```python
from build123d import *

# Parameters (mm, degrees)
EXTRUDE1_DEPTH          = 12.7
F_1_4_CLEARANCE_HOLE1_D = 7.14248
CHAMFER1_SIZE           = 4.7625


with BuildPart() as part:
    # Sketch1 → Extrude1 (new, symmetric)
    with BuildSketch(Plane.XY):
        with BuildLine():
            Line((22.225, 26.9875), (0.79375, 26.9875))
            Line((0.79375, 26.9875), (0.79375, 12.675171042))
            ThreePointArc((0.79375, 12.675171042), (0, -12.7), (-0.79375, 12.675171042))
            Line((-0.79375, 12.675171042), (-0.79375, 26.9875))
            Line((-0.79375, 26.9875), (-22.225, 26.9875))
            Line((-22.225, 26.9875), (-22.225, -30.1625))
            Line((-22.225, -30.1625), (-41.275, -30.1625))
            Line((-41.275, -30.1625), (-41.275, -38.1))
            Line((-41.275, -38.1), (41.275, -38.1))
            Line((41.275, -38.1), (41.275, -30.1625))
            Line((41.275, -30.1625), (22.225, -30.1625))
            Line((22.225, -30.1625), (22.225, 26.9875))
        make_face()
    extrude(amount=EXTRUDE1_DEPTH, both=True)

    # 1/4 Clearance Hole1 (through all)
    with Locations(Plane.XZ.offset(38.1)):
        with Locations((-31.75, 0), (31.75, 0)):
            Hole(F_1_4_CLEARANCE_HOLE1_D / 2)

    # Chamfer1
    chamfer1_edges = [part.edges().sort_by_distance(p)[0] for p in [
        (-22.225, 26.9875, 0),
        (22.225, 26.9875, 0),
    ]]
    chamfer(chamfer1_edges, length=CHAMFER1_SIZE)


solid = part.part
```
Can you work these out from the model? Positions are in its coordinate system, mm. A direction names the side the tool comes from. Coordinates: 2 decimals unless noted, no trailing zeros. Loops run counter-clockwise (first coordinate to the right, second up) from the corner with the lowest first, then second, coordinate; pieces in that order, holes last. Notation, with made-up numbers: M -33.5,-12 L -11.5,-12 A8 cw -11.5,-8 Z; hole C 3.25,82.25 d1. An arc over 180 degrees is marked long. Put each result on its own line as item: value. Start each with the question number.
(1) We'd pull the mould along Z, two halves only. Please class faces 5 (the face through (-35.156, -34.076, 1.073)), 6 (the face through (28.344, -34.076, 1.073)), 7 (the face through (-10, -12, 12.7)), 8 (the face through (-41.275, -34, 0)): +Z half, -Z half, draft (parallel to the pull), parting line (faces both ways), or undercut.
(2) Imagine slicing it at C-C on y = 0. List the corners of the cut face in (x, z) for me (3 decimals), and give its area (3 significant figures).
(3) Imagine slicing it at A-A on x = 31.75. List the corners of the cut face in (y, z) for me.
(4) Imagine slicing it at B-B on z = 0. List the corners of the cut face in (x, y) for me (1 decimal).
(5) I need wall thicknesses on probe 1 along Z at (x, y) = (31.75, -35.25); probe 2 along X at (y, z) = (0, -3.5) (3 decimals); probe 3 along X at (y, z) = (13, -4.25) (3 decimals). Which ranges of each line are inside material? Lowest first, please.
(6) Imagine slicing it at D-D on z = -6. List the corners of the cut face in (x, y) for me (1 decimal).
(7) Will these pins go through, and if not, where does the flat tip stop? pin 1 Ø15 at (x, z) = (31.5, -0.5) entering from +Y; pin 2 Ø4 at (y, z) = (18.5, -7.5) entering from +X (3 decimals); pin 3 Ø7 at (y, z) = (22, -5.5) entering from -X (3 decimals).
(8) Which directions (+Z, -Z, +X, -X, +Y, -Y) give clear straight access to the entire face, cutting with the end or side of a thin tool? Please do faces 1 (the face through (22.225, -4, 0)), 2 (the face through (-0.794, 20, 0)), 3 (the face through (-10, -12, -12.7)), 4 (the face through (-22.225, -4, 0)).
Worked answers:
1. face 5: undercut
1. face 6: undercut
1. face 7: +Z half
1. face 8: draft
2. outline: M -22.225,-12.7 L -12.7,-12.7 L -12.7,12.7 L -22.225,12.7 Z; M 12.7,-12.7 L 22.225,-12.7 L 22.225,12.7 L 12.7,12.7 Z
2. area: 484 mm2
3. outline: M -38.1,-12.7 L -30.16,-12.7 L -30.16,-3.57 L -38.1,-3.57 Z; M -38.1,3.57 L -30.16,3.57 L -30.16,12.7 L -38.1,12.7 Z
4. outline: M -41.3,-38.1 L -35.3,-38.1 L -35.3,-30.2 L -41.3,-30.2 Z; M -28.2,-38.1 L 28.2,-38.1 L 28.2,-30.2 L 22.2,-30.2 L 22.2,22.2 L 17.5,27 L 0.8,27 L 0.8,12.7 A12.7 cw long -0.8,12.7 L -0.8,27 L -17.5,27 L -22.2,22.2 L -22.2,-30.2 L -28.2,-30.2 Z; M 35.3,-38.1 L 41.3,-38.1 L 41.3,-30.2 L 35.3,-30.2 Z
5. probe 1: z = -12.7 to -3.57, 3.57 to 12.7
5. probe 2: x = -22.225 to -12.7, 12.7 to 22.225
5. probe 3: x = -22.225 to -0.794, 0.794 to 22.225
6. outline: M -41.3,-38.1 L 41.3,-38.1 L 41.3,-30.2 L 22.2,-30.2 L 22.2,22.2 L 17.5,27 L 0.8,27 L 0.8,12.7 A12.7 cw long -0.8,12.7 L -0.8,27 L -17.5,27 L -22.2,22.2 L -22.2,-30.2 L -41.3,-30.2 Z
7. pin 1: stops at y = -30.16
7. pin 2: stops at x = 22.225
7. pin 3: stops at x = -22.225
8. face 1: +Z, -Z, +X, +Y
8. face 2: +Z, -Z, +Y
8. face 3: -Z, +X, -X, +Y, -Y
8. face 4: +Z, -Z, -X, +Y
